Input: part model. Units: mm. Frame: model coordinates. Coordinates: 2 decimals unless noted, no trailing zeros. Loops run counter-clockwise (first coordinate to the right, second up) from the corner with the lowest first, then second, coordinate; pieces in that order, holes last.
```python
from build123d import *

# Parameters (mm, degrees)
SKETCH_1_W      = 68
SKETCH_1_H      = 50
SKETCH_1_R      = 2.5
EXTRUDE_1_DEPTH = 1.5


with BuildPart() as part:
    # ｽｹｯﾁ1 → ﾎﾞｽ - 押し出し1 (new body)
    with BuildSketch(Plane.XY):
        Rectangle(SKETCH_1_W, SKETCH_1_H)
        with Locations((-29, 0)):
            Circle(SKETCH_1_R, mode=Mode.SUBTRACT)
        with Locations(Location((29, 0, 0), (0, 0, 180))):
            Circle(SKETCH_1_R, mode=Mode.SUBTRACT)
    extrude(amount=EXTRUDE_1_DEPTH)


solid = part.part
```
Item 1: Line query: L1, parallel to Y at x = 29, z = 0.6; L2, parallel to X at y = 2, z = 1.05; L3, parallel to Y at x = -30, z = 0.65. Output: solid intervals per line, ascending.
Result:
L1: y = -25 to -2.5, 2.5 to 25
L2: x = -34 to -30.5, -27.5 to 27.5, 30.5 to 34
L3: y = -25 to -2.29, 2.29 to 25
Item 2: Section query A-A (x = -29). Output: boundary loops of the cut face in (y, z), then the cut area to 3 significant figures.
Result:
outline: (-25, 0) - (-2.5, 0) - (-2.5, 1.5) - (-25, 1.5) - close; (2.5, 0) - (25, 0) - (25, 1.5) - (2.5, 1.5) - close
area: 67.5 mm2
Item 3: Contact query for a flat-ended pin moving along its axis: P1, Ø3, axis at x = 29, y = 0, coming from the -Z side. Output: stop coordinate, or through.
Result:
P1: passes through
Item 4: Mould query, pull axis X, two halves, no side actions, for faces 1 (the face through (31.5, -0.1, 0.7)), 2 (the face through (0, 25, 1)), 3 (the face through (34, 0, 1)), 4 (the face through (-31.5, 0.1, 0.7)). Classes: +X half, -X half, draft (parallel to the pull), parting line (faces both ways), or undercut.
Result:
face 1: undercut
face 2: draft
face 3: +X half
face 4: undercut
Item 5: Section query B-B (y = 1). Output: boundary loops of the cut face in (x, z).
Result:
outline: (-34, 0) - (-31.29, 0) - (-31.29, 1.5) - (-34, 1.5) - close; (-26.71, 0) - (26.71, 0) - (26.71, 1.5) - (-26.71, 1.5) - close; (31.29, 0) - (34, 0) - (34, 1.5) - (31.29, 1.5) - close
